Could you check a few things on this model? Use its own coordinates, in mm. Round coordinates to 2 decimals unless told otherwise and drop trailing zeros. Order: outer loops, then holes, each group sorted by start corner. A loop starts at its lowest first (then second) coordinate and runs counter-clockwise, first axis right, second up. Notation, with made-up numbers: (48.25, 25.5) - (96.25, 25.5) arc R15 ccw to (96.25, 35.5) - close; hole circle Ø5 at (77.25, 66). An arc over 180 degrees is marked (long way). Use one line per item in the form item = value.
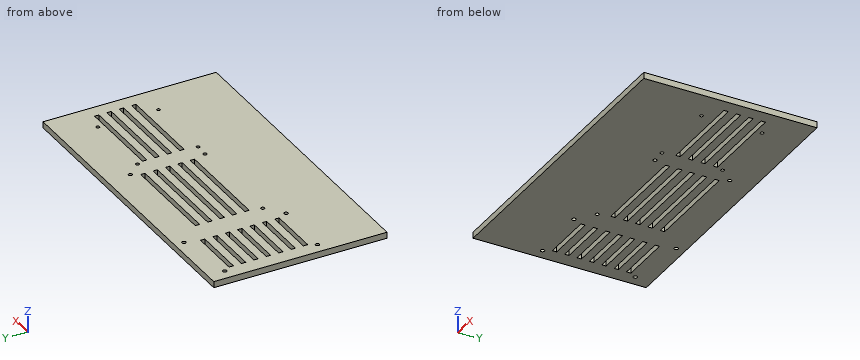
from build123d import *

# Parameters (mm, degrees)
CROQUIS1_W              = 250
CROQUIS1_H              = 140
CROQUIS1_R              = 1.6
CROQUIS1_R_2            = 1.375
CROQUIS1_R_3            = 1.5
CROQUIS1_W_2            = 41.859919993
CROQUIS1_H_2            = 3.5
CROQUIS1_W_3            = 79.963180499
CROQUIS1_W_4            = 70.346682928
SALIENTE_EXTRUIR1_DEPTH = 5


with BuildPart() as part:
    # Croquis1 → Saliente-Extruir1 (new body)
    with BuildSketch(Plane.XY):
        with Locations((14.354712009, 16.335108086)):
            Rectangle(CROQUIS1_W, CROQUIS1_H)
        with Locations((-101.706636686, -2.394891914)):
            Circle(CROQUIS1_R, mode=Mode.SUBTRACT)
        with Locations((-53.446636686, -3.664891914)):
            Circle(CROQUIS1_R, mode=Mode.SUBTRACT)
        with Locations((114.247224856, 6.848582104)):
            Circle(CROQUIS1_R_2, mode=Mode.SUBTRACT)
        with Locations((114.247224856, 55.848582104)):
            Circle(CROQUIS1_R_2, mode=Mode.SUBTRACT)
        with Locations((56.247224856, 6.848582104)):
            Circle(CROQUIS1_R_2, mode=Mode.SUBTRACT)
        with Locations((56.247224856, 55.848582104)):
            Circle(CROQUIS1_R_2, mode=Mode.SUBTRACT)
        with Locations((46.159209602, 67.214416737)):
            Circle(CROQUIS1_R_3, mode=Mode.SUBTRACT)
        with Locations((45.159209602, 7.414416737)):
            Circle(CROQUIS1_R_3, mode=Mode.SUBTRACT)
        with Locations((-39.460790398, 7.414416737)):
            Circle(CROQUIS1_R_3, mode=Mode.SUBTRACT)
        with Locations((-101.706636686, 72.535108086)):
            Circle(CROQUIS1_R, mode=Mode.SUBTRACT)
        with Locations((-53.446636686, 78.885108086)):
            Circle(CROQUIS1_R, mode=Mode.SUBTRACT)
        with Locations((-77.501473664, 55.441697687)):
            Rectangle(CROQUIS1_W_2, CROQUIS1_H_2, mode=Mode.SUBTRACT)
        with Locations((-77.501473664, 65.441697687)):
            Rectangle(CROQUIS1_W_2, CROQUIS1_H_2, mode=Mode.SUBTRACT)
        with Locations((-77.501473664, 45.441697687)):
            Rectangle(CROQUIS1_W_2, CROQUIS1_H_2, mode=Mode.SUBTRACT)
        with Locations((-77.501473664, 35.441697687)):
            Rectangle(CROQUIS1_W_2, CROQUIS1_H_2, mode=Mode.SUBTRACT)
        with Locations((-77.501473664, 25.441697687)):
            Rectangle(CROQUIS1_W_2, CROQUIS1_H_2, mode=Mode.SUBTRACT)
        with Locations((-77.501473664, 15.441697687)):
            Rectangle(CROQUIS1_W_2, CROQUIS1_H_2, mode=Mode.SUBTRACT)
        with Locations((-77.501473664, 5.441697687)):
            Rectangle(CROQUIS1_W_2, CROQUIS1_H_2, mode=Mode.SUBTRACT)
        with Locations((2.730039656, 48.964416737)):
            Rectangle(CROQUIS1_W_3, CROQUIS1_H_2, mode=Mode.SUBTRACT)
        with Locations((2.730039656, 58.964416737)):
            Rectangle(CROQUIS1_W_3, CROQUIS1_H_2, mode=Mode.SUBTRACT)
        with Locations((2.730039656, 38.964416737)):
            Rectangle(CROQUIS1_W_3, CROQUIS1_H_2, mode=Mode.SUBTRACT)
        with Locations((2.730039656, 28.964416737)):
            Rectangle(CROQUIS1_W_3, CROQUIS1_H_2, mode=Mode.SUBTRACT)
        with Locations((2.730039656, 18.964416737)):
            Rectangle(CROQUIS1_W_3, CROQUIS1_H_2, mode=Mode.SUBTRACT)
        with Locations((93.196116464, 38.964416737)):
            Rectangle(CROQUIS1_W_4, CROQUIS1_H_2, mode=Mode.SUBTRACT)
        with Locations((93.196116464, 48.964416737)):
            Rectangle(CROQUIS1_W_4, CROQUIS1_H_2, mode=Mode.SUBTRACT)
        with Locations((93.196116464, 28.964416737)):
            Rectangle(CROQUIS1_W_4, CROQUIS1_H_2, mode=Mode.SUBTRACT)
        with Locations((93.196116464, 18.964416737)):
            Rectangle(CROQUIS1_W_4, CROQUIS1_H_2, mode=Mode.SUBTRACT)
    extrude(amount=SALIENTE_EXTRUIR1_DEPTH)


solid = part.part
Item 1: Will these pins go through, and if not, where does the flat tip stop? P1, Ø8, axis at x = -61, y = 69, coming from the -Z side; P2, Ø1.9, axis at x = -53.45, y = 78.89, coming from the -Z side.
Found:
P1 = 0
P2 = through
Item 2: I need wall thicknesses on L1, parallel to Y at x = -11.5, z = 1.6; L2, parallel to X at y = 49, z = 1.85; L3, parallel to Y at x = 124, z = 2.9. Which ranges of each line are inside material? Lowest first, please.
Found:
L1 = -53.66 to 17.21, 20.71 to 27.21, 30.71 to 37.21, 40.71 to 47.21, 50.71 to 57.21, 60.71 to 86.34
L2 = -110.65 to -37.25, 42.71 to 58.02, 128.37 to 139.35
L3 = -53.66 to 17.21, 20.71 to 27.21, 30.71 to 37.21, 40.71 to 47.21, 50.71 to 86.34
Item 3: Imagine slicing it at A-A on x = -34. Please give me the cut outline in (y, z), plus the area to 4 significant figures.
Found:
outline = (-53.66, 0) - (17.21, 0) - (17.21, 5) - (-53.66, 5) - close; (20.71, 0) - (27.21, 0) - (27.21, 5) - (20.71, 5) - close; (30.71, 0) - (37.21, 0) - (37.21, 5) - (30.71, 5) - close; (40.71, 0) - (47.21, 0) - (47.21, 5) - (40.71, 5) - close; (50.71, 0) - (57.21, 0) - (57.21, 5) - (50.71, 5) - close; (60.71, 0) - (86.34, 0) - (86.34, 5) - (60.71, 5) - close
area = 612.5 mm2
Item 4: Imagine slicing it at B-B on x = -87.5. State how many separate pieces and enclosed holes the cut face has, plus the area to 4 significant figures.
Found:
separate_pieces = 8
enclosed_holes = 0
area = 577.5 mm2
